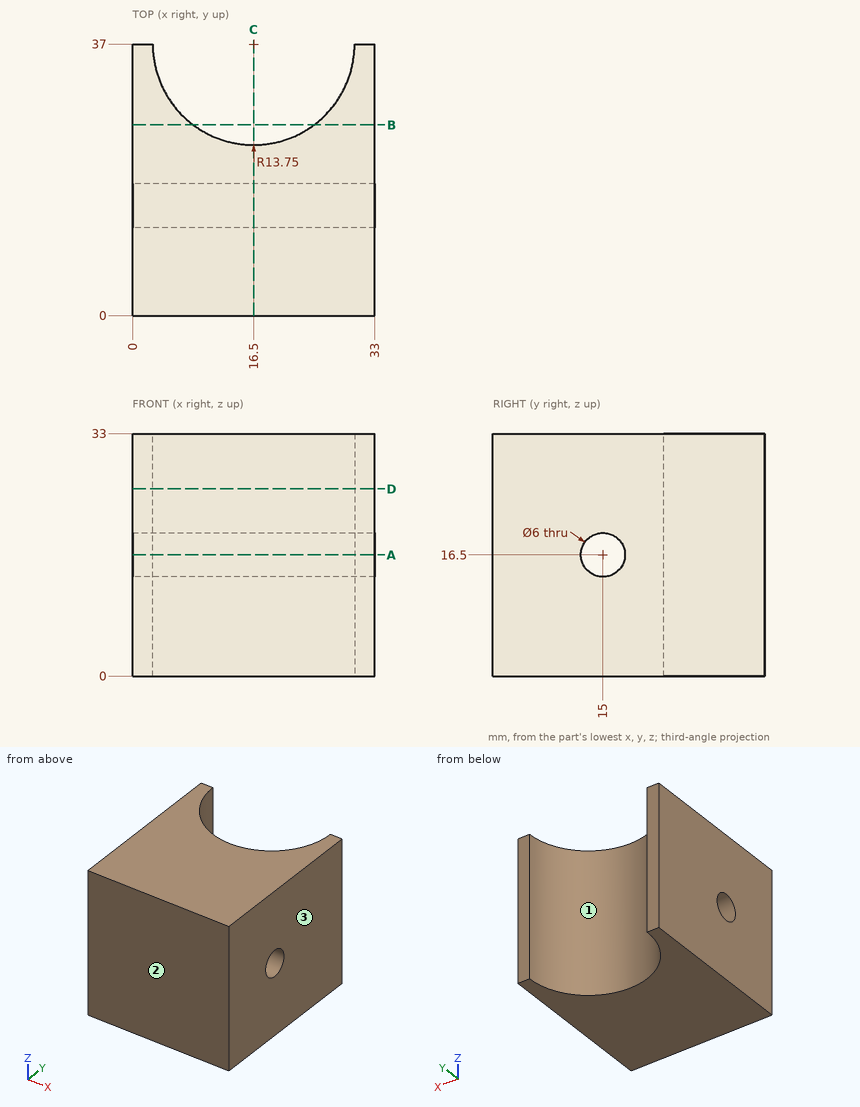
Study the drawing (mm; zero at the part's minimum x, y, z) and answer. Give positions to 0.01 mm unless a question says otherwise; leave off trailing zeros. Write each loop counter-clockwise with the first axis right and the second up, starting at its lowest first coordinate (ties: lowest second). Pieces come first, ordered by that corner, then holes. Notation, with made-up numbers: (87.5, 24) -> (124.5, 24) arc R20 cw to (124.5, 32) -> close; hole circle Ø7 at (87.25, -16). An arc over 180 degrees is marked (long way). Write item = value, one per line. Start each with the question number.
1) This flat-tipped pin is pushed along its axis until it touches: pin 1 (10 mm diameter, centred on x = 24, z = 20, fed in from +Y). Where does it stop, or does it pass through?
2) The part is cut by section C-C, the plane x = 16.5. Determine the outline of the cut face in (y, z), and give its area (3 significant figures).
3) The part is cut by section D-D, the plane z = 25.5. Determine the outline of the cut face in (x, y).
4) Determine the mould class of the marked faces 1, 2 and 3 for opening direction X: +X half, -X half, draft (parallel to the pull), parting line (faces both ways), or undercut.
5) Straight lines are drawn through the part: line 1 along Y through (x, z) = (16, 16.5); line 2 along Z through (x, y) = (26, 15.5); line 3 along Y through (x, z) = (14, 17.5). For each, find the intervals that lie inside material, in ascending order.
6) The part is cut by section B-B, the plane y = 26. Determine the outline of the cut face in (x, z), and give its area (4 significant figures).
7) The part is cut by section A-A, the plane z = 16.5. Determine the outline of the cut face in (x, y).
Solutions:
q1.pin_1 = 31.27
q2.outline = (0, 0) -> (23.25, 0) -> (23.25, 33) -> (0, 33) -> close; hole circle Ø6 at (15, 16.5)
q2.area = 739 mm²
q3.outline = (0, 0) -> (33, 0) -> (33, 37) -> (30.25, 37) arc R13.75 cw to (2.75, 37) -> (0, 37) -> close
q4.face_1 = undercut
q4.face_2 = draft
q4.face_3 = +X half
q5.line_1 = 0 to 12, 18 to 23.26
q5.line_2 = 0 to 13.54, 19.46 to 33
q5.line_3 = 0 to 12.17, 17.83 to 23.48
q6.outline = (0, 0) -> (8.25, 0) -> (8.25, 33) -> (0, 33) -> close; (24.75, 0) -> (33, 0) -> (33, 33) -> (24.75, 33) -> close
q6.area = 544.5 mm²
q7.outline = (0, 0) -> (33, 0) -> (33, 12) -> (0, 12) -> close; (0, 18) -> (33, 18) -> (33, 37) -> (30.25, 37) arc R13.75 cw to (2.75, 37) -> (0, 37) -> close
